```python
from build123d import *

# Parameters (mm, degrees)
IZIM2_R                     = 28
Y_KSEKLIK_EKSTR_ZYON5_DEPTH = 10
IZIM3_R                     = 1.49
KES_EKSTR_ZYON1_DEPTH       = 54.801017528
DAIRESEL_KAPLAMA1_COUNT     = 4
IZIM4_R                     = 3
IZIM4_R_2                   = 1.6
Y_KSEKLIK_EKSTR_ZYON6_DEPTH = 3
DAIRESEL_KAPLAMA2_COUNT     = 4


with BuildPart() as part:
    # izim2 → Y_kseklik-Ekstr_zyon5 (new body)
    with BuildSketch(Plane(origin=(0, 0, 0), x_dir=(1, 0, 0), z_dir=(0, 1, 0))):
        with BuildLine():
            ThreePointArc((-37.380138356, -2.867988228), (-36.240115286, -9.599694998), (-33.898134186, -16.013013418))
            ThreePointArc((-33.898134186, -16.013013418), (-28.838645946, -16.65), (-30.816743504, -21.350138636))
            ThreePointArc((-30.816743504, -21.350138636), (-18.652225356, -32.52067941), (-2.867988228, -37.380138356))
            ThreePointArc((-2.867988228, -37.380138356), (0, -33.5), (2.867988228, -37.380138356))
            ThreePointArc((2.867988228, -37.380138356), (18.652225356, -32.52067941), (30.816743504, -21.350138636))
            ThreePointArc((30.816743504, -21.350138636), (28.838645946, -16.65), (33.898134186, -16.013013418))
            ThreePointArc((33.898134186, -16.013013418), (36.240115286, -9.599694998), (37.380138356, -2.867988228))
            ThreePointArc((37.380138356, -2.867988228), (33.5, 0), (37.380138356, 2.867988228))
            ThreePointArc((37.380138356, 2.867988228), (36.240115286, 9.599694998), (33.898134186, 16.013013418))
            ThreePointArc((33.898134186, 16.013013418), (28.838645946, 16.65), (30.816743504, 21.350138636))
            ThreePointArc((30.816743504, 21.350138636), (18.652225356, 32.52067941), (2.867988228, 37.380138356))
            ThreePointArc((2.867988228, 37.380138356), (0, 33.5), (-2.867988228, 37.380138356))
            ThreePointArc((-2.867988228, 37.380138356), (-18.652225356, 32.52067941), (-30.816743504, 21.350138636))
            ThreePointArc((-30.816743504, 21.350138636), (-28.838645946, 16.65), (-33.898134186, 16.013013418))
            ThreePointArc((-33.898134186, 16.013013418), (-36.240115286, 9.599694998), (-37.380138356, 2.867988228))
            ThreePointArc((-37.380138356, 2.867988228), (-33.5, 0), (-37.380138356, -2.867988228))
        make_face()
        with Locations(Location((0, 0, 0), (0, 0, 270))):
            Circle(IZIM2_R, mode=Mode.SUBTRACT)
    extrude(amount=Y_KSEKLIK_EKSTR_ZYON5_DEPTH)

    # izim3 → Kes-Ekstr_zyon1 (cut, through all)
    with BuildSketch(Plane(origin=(0, 0, 0), x_dir=(0.7071067811865464, 0, 0.7071067811865488), z_dir=(-0.7071067811865488, 0, 0.7071067811865464))):
        with Locations((0, 5)):
            Circle(IZIM3_R)
    kes_ekstr_zyon1 = extrude(amount=-KES_EKSTR_ZYON1_DEPTH, mode=Mode.SUBTRACT)

    # Dairesel Kaplama1: Kes-Ekstr_zyon1 ×4 about axis
    dairesel_kaplama1_axis = Axis((0, 31.917325532, 0), (0, -1, 0))
    for i in range(1, DAIRESEL_KAPLAMA1_COUNT):
        add(kes_ekstr_zyon1.rotate(dairesel_kaplama1_axis, i * 360 / DAIRESEL_KAPLAMA1_COUNT), mode=Mode.SUBTRACT)

    # izim4 → Y_kseklik-Ekstr_zyon6 (add)
    with BuildSketch(Plane(origin=(0, 0, 0), x_dir=(1, 0, 0), z_dir=(0, 1, 0))):
        with Locations((-36.5, 0)):
            Circle(IZIM4_R)
        with Locations(Location((-36.5, 0, 0), (0, 0, 270))):
            Circle(IZIM4_R_2, mode=Mode.SUBTRACT)
    y_kseklik_ekstr_zyon6 = extrude(amount=Y_KSEKLIK_EKSTR_ZYON6_DEPTH)

    # Dairesel Kaplama2: Y_kseklik-Ekstr_zyon6 ×4 about axis
    dairesel_kaplama2_axis = Axis((0, 0, 0), (0, 1, 0))
    for i in range(1, DAIRESEL_KAPLAMA2_COUNT):
        add(y_kseklik_ekstr_zyon6.rotate(dairesel_kaplama2_axis, i * 360 / DAIRESEL_KAPLAMA2_COUNT))


solid = part.part
```
Model file for the job. Use its own axes, mm. A direction names the side the tool comes from. Coordinates: 2 decimals unless noted, no trailing zeros. Write each loop counter-clockwise with the first axis right and the second up, starting at its lowest first coordinate (ties: lowest second). Pieces come first, ordered by that corner, then holes. Notation, with made-up numbers: (80.5, 18.5) - (108.5, 18.5) arc R22 ccw to (108.5, 32.5) - close; hole circle Ø10 at (-2.5, -6). An arc over 180 degrees is marked (long way). One line per question, with ' | ' between items. Start each with the question number.
Q1. Pin check, flat tips, straight feed: pin 1 (5 mm diameter, centred on y = 8, z = -22.5, fed in from -X); pin 2 (1.5 mm diameter, centred on x = 19.5, y = 7, fed in from -Z); pin 3 (3 mm diameter, centred on y = 5, z = -9, fed in from -X). Stop position of each tip, or through.
Q2. 3-axis set-ups, long thin cutter, end or side, ignore diameter. For faces 5 (the face through (-37.92, 1.48, 0.74)), 6 (the face through (33.5, 6.5, 0.1)): which of +Z, -Z, +X, -X, +Y, -Y reach the whole face in a straight line?
Q3. Cut at B-B, the plane z = -8. List the corners of the cut face in (x, y), then the cut area to 3 significant figures.
Q4. Cut at C-C, the plane z = 4. List the corners of the cut face in (x, y).
Q5. Drill centre lines: line 1 (X direction, y = 1.05, z = 0); line 2 (X direction, y = 5.5, z = 0); line 3 (X direction, y = 5.25, z = 24). Where is each one in solid material? Low to high. Write a range as [from, to].
Q6. Pull direction Y, two halves, no side cores. Call faces 1 (the face through (-22.09, 5.45, -24.1)), 2 (the face through (22.956, 6.477, -23.23)), 3 (the face through (0.1, 6.5, -33.5)), 4 (the face through (35, 3, -1)): pulls with the +Y half, pulls with the -Y half, needs draft (parallel to the pull), parting line crosses it, or undercut.
Q7. Cut at A-A, the plane x = 0. List the corners of the cut face in (y, z), then the cut area to 3 significant figures.
Answer below:
1) pin 1: x = -30.82 | pin 2: z = -32.46 | pin 3: x = -36.73
2) face 5: +Y, -Y | face 6: +Y
3) outline: (-36.63, 0) - (-26.83, 0) - (-26.83, 10) - (-36.63, 10) - close; (26.83, 0) - (36.63, 0) - (36.63, 10) - (26.83, 10) - close | area: 196 mm^2
4) outline: (-37.28, 0) - (-27.71, 0) - (-27.71, 10) - (-37.28, 10) - close; (27.71, 0) - (37.28, 0) - (37.28, 10) - (27.71, 10) - close
5) line 1: [-39.5, -38.1], [-34.9, -28], [28, 34.9], [38.1, 39.5] | line 2: [-33.5, -28], [28, 33.5] | line 3: [-28.8, -26.08], [-21.92, -14.42], [14.42, 21.92], [26.08, 28.8]
6) face 1: undercut | face 2: undercut | face 3: needs draft | face 4: pulls with the +Y half
7) outline: (0, -39.5) - (3, -39.5) - (3, -38.1) - (0, -38.1) - close; (0, -34.9) - (3, -34.9) - (3, -33.5) - (10, -33.5) - (10, -28) - (0, -28) - close; (0, 28) - (10, 28) - (10, 33.5) - (3, 33.5) - (3, 34.9) - (0, 34.9) - close; (0, 38.1) - (3, 38.1) - (3, 39.5) - (0, 39.5) - close | area: 127 mm^2
